The drawing under review shows one solid part. Ordinate dimensions are in mm from its lowest x, y, z. Give positions to 0.01 mm unless a question says otherwise; leave off trailing zeros. Order: outer loops, then holes, each group sorted by start corner. A loop starts at its lowest first (then second) coordinate and runs counter-clockwise, first axis right, second up. Notation, with made-up numbers: (14, 67.25) - (57, 67.25) arc R33 ccw to (57, 97.25) - close; hole circle Ø3 at (55, -35.75). An arc over 180 degrees is marked (long way). Use CSV: the item, a comma, the result in double quotes. Start each with the question number.
1. Take a section at A-A, the plane x = 6.35. State the section outline as (y, z) points (1 decimal).
2. Take a section at C-C, the plane z = 4.75. State the section outline as (x, y) points, then the cut area to 3 significant figures.
3. To check wall thickness, follow line 1 (Y direction, x = 6.35, z = 1.15); line 2 (X direction, y = 5.25, z = 3.5); line 3 (Z direction, x = 4.25, y = 3) (3 decimals). State the ranges of each line that lie inside material, in increasing order. Write a range as [from, to].
4. Take a section at D-D, the plane z = 1. State the section outline as (x, y) points.
5. Draft analysis for pull direction Y (two halves, no side actions). For the marked faces 1, 2 and 3, state which applies: released by +Y, released by -Y, zero draft, split by the parting line, or undercut.
6. For pin 1 (3 mm diameter, centred on y = 11, z = 3.5, fed in from -X), flat-tipped, find the tip position at first contact; note if it passes through.
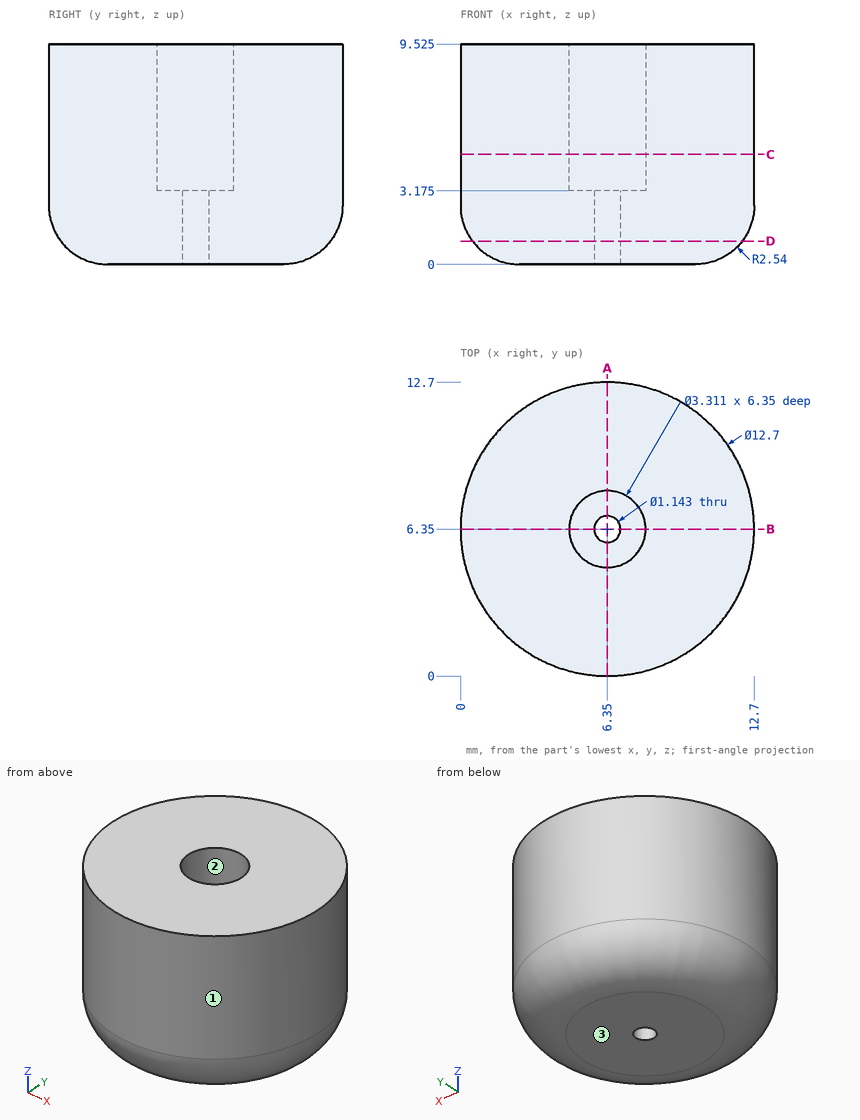
Determined:
1,outline,"(0, 2.5) arc R2.5 ccw to (2.5, 0) - (5.8, 0) - (5.8, 3.2) - (4.7, 3.2) - (4.7, 9.5) - (0, 9.5) - close; (6.9, 0) - (10.2, 0) arc R2.5 ccw to (12.7, 2.5) - (12.7, 9.5) - (8, 9.5) - (8, 3.2) - (6.9, 3.2) - close"
2,outline,"circle Ø12.7 at (6.35, 6.35); hole circle Ø3.31 at (6.35, 6.35)"
2,area,"118 mm²"
3,line 1,"y = [0.41, 5.78], [6.92, 12.29]"
3,line 2,"x = [0.1, 5.11], [7.59, 12.6]"
3,line 3,"z = [0.004, 9.525]"
4,outline,"circle Ø11.66 at (6.35, 6.35); hole circle Ø1.14 at (6.35, 6.35)"
5,face 1,"split by the parting line"
5,face 2,"undercut"
5,face 3,"zero draft"
6,pin 1,"stops at x = 0.84"
